Source: CAD feature listing. Evaluate the final solid. Frame: model axes, mm. A direction names the side the tool comes from. Give positions to 0.01 mm unless a question says otherwise; leave off trailing zeros. Order: outer loops, then holes, each group sorted by start corner. A loop starts at its lowest first (then second) coordinate and runs counter-clockwise, first axis right, second up. Notation, with made-up numbers: (67, -25.5) - (95, -25.5) arc R30 ccw to (95, 9.5) - close; hole circle Ø1 at (-20, 23.5). An arc over 180 degrees is marked (long way). Answer as CSV lines item,"result".
```python
from build123d import *

# Parameters (mm, degrees)
F0_R     = 36.130813
F1_DEPTH = 3
F2_R     = 26.349485
F3_DEPTH = 25.4
F4_R     = 13.809058
F5_DEPTH = 25.4
F6_SIZE  = 0.5


with BuildPart() as f1:
    # F0 (on Top) → F1 (new body)
    with BuildSketch(Plane.XY):
        Circle(F0_R)
    extrude(amount=F1_DEPTH)

    # F2 (on Top) → F3 (join)
    with BuildSketch(Plane.XY):
        Circle(F2_R)
    extrude(amount=F3_DEPTH)

    # F4 (on face) → F5 (join)
    with BuildSketch(Plane.XY.offset(25.4)):
        Circle(F4_R)
    extrude(amount=F5_DEPTH)

    # F6
    f6_edges = [f1.edges().sort_by_distance(p)[0] for p in [
        (-26.349485, 0, 25.4),
    ]]
    chamfer(f6_edges, length=F6_SIZE)


solid = f1.part
```
(1) Cut plane A-A (x = 0). Return loops of the section in (y, z), then the cut area to 3 significant figures.
Completed:
outline,"(-36.13, 0) - (36.13, 0) - (36.13, 3) - (26.35, 3) - (26.35, 24.9) - (25.85, 25.4) - (13.81, 25.4) - (13.81, 50.8) - (-13.81, 50.8) - (-13.81, 25.4) - (-25.85, 25.4) - (-26.35, 24.9) - (-26.35, 3) - (-36.13, 3) - close"
area,"2,100 mm²"
(2) Cut plane D-D (z = 31.5). Return loops of the section in (x, y), then the cut area to 3 significant figures.
Completed:
outline,"circle Ø27.62 at (0, 0)"
area,"599 mm²"
(3) Contact query for flat-ended pins moving along their axis: pin 1 (5 mm diameter, centred on x = 2.5, z = 25.5, fed in from -Y); pin 2 (5 mm diameter, centred on x = 18, y = -14, fed in from +Z); pin 3 (3 mm diameter, centred on x = -17, z = 26.5, fed in from -Y). Output: stop coordinate, or through.
Completed:
pin 1,"y = -26.35"
pin 2,"z = 25.4"
pin 3,"y = -20.36"
(4) Cut plane C-C (z = 16.5). Return loops of the section in (x, y), then the cut area to 3 significant figures.
Completed:
outline,"circle Ø52.7 at (0, 0)"
area,"2,180 mm²"
(5) Access query for faces 1 (the flat face through (11, -11, 25.4)), 2 (the flat face through (0, 0, 50.8)). Directions: +Z, -Z, +X, -X, +Y, -Y. A direction counts if a zero-diameter tool reaches every point of the face in a straight line with its end or side. Return the directions, or none.
Completed:
face 1,"+Z"
face 2,"+Z, +X, -X, +Y, -Y"
(6) Ray query, line 1 (Z direction, x = 1.5, y = 16.5); line 2 (Y direction, x = 0, z = 10); line 3 (Z direction, x = 10, y = 31). Return the intervals inside material, ascending. Write a range as from..to.
Completed:
line 1,"0..25.4"
line 2,"-26.35..26.35"
line 3,"0..3"
